from build123d import *

# Parameters (mm, degrees)
EXTRUDE_1_DEPTH     = 6
FILLET_1_R          = 0.5
SKETCH_2_W          = 0.4
SKETCH_2_H          = 0.4
EXTRUDE_2_DEPTH     = 2.5
SKETCH_3_W          = 0.8
SKETCH_3_H          = 5.4
CUT_EXTRUDE_1_DEPTH = 0.5
SKETCH_4_W          = 0.8
SKETCH_4_H          = 5.4
CUT_EXTRUDE_2_DEPTH = 0.5
SKETCH_5_W          = 0.5
SKETCH_5_H          = 4
CUT_EXTRUDE_3_DEPTH = 0.5
SKETCH_6_W          = 0.5
SKETCH_6_H          = 4
CUT_EXTRUDE_4_DEPTH = 0.5
SKETCH_7_R          = 0.35
EXTRUDE_3_DEPTH     = 0.7


with BuildPart() as part:
    # 草图1 → 凸台-拉伸1 (new body)
    with BuildSketch(Plane.XY):
        Polygon((-7, 5), (-2.5, 5), (-2.5, -2.5), (2.5, -2.5), (2.5, 5), (7, 5), (7, -5), (-7, -5), align=None)
    extrude(amount=EXTRUDE_1_DEPTH)

    # 圆角1
    fillet_1_edges = [part.edges().sort_by_distance(p)[0] for p in [
        (-2.5, 5, 3),
        (2.5, 5, 3),
    ]]
    fillet(fillet_1_edges, radius=FILLET_1_R)

    # 草图2 → 凸台-拉伸2 (add)
    with BuildSketch(Plane.XZ.offset(5)):
        with Locations((-5.15, 4.27)):
            Rectangle(SKETCH_2_W, SKETCH_2_H)
        with Locations((5.15, 4.27)):
            Rectangle(SKETCH_2_W, SKETCH_2_H)
        with Locations((-5.15, 1.73)):
            Rectangle(SKETCH_2_W, SKETCH_2_H)
        with Locations((5.15, 1.73)):
            Rectangle(SKETCH_2_W, SKETCH_2_H)
    extrude(amount=EXTRUDE_2_DEPTH)

    # 草图3 → 切除-拉伸1 (cut)
    with BuildSketch(Plane.ZY.offset(7)):
        with Locations((3.003385533, 2.3)):
            Rectangle(SKETCH_3_W, SKETCH_3_H)
    extrude(amount=-CUT_EXTRUDE_1_DEPTH, mode=Mode.SUBTRACT)

    # 草图4 → 切除-拉伸2 (cut)
    with BuildSketch(Plane(origin=(7, 0, 0), x_dir=(0, 0, -1), z_dir=(1, 0, 0))):
        with Locations((-3.003385533, 2.3)):
            Rectangle(SKETCH_4_W, SKETCH_4_H)
    extrude(amount=-CUT_EXTRUDE_2_DEPTH, mode=Mode.SUBTRACT)

    # 草图5 → 切除-拉伸3 (cut)
    with BuildSketch(Plane(origin=(-2.5, 0, 0), x_dir=(0, 0, -1), z_dir=(1, 0, 0))):
        with Locations((-3.003385533, 3)):
            Rectangle(SKETCH_5_W, SKETCH_5_H)
    extrude(amount=-CUT_EXTRUDE_3_DEPTH, mode=Mode.SUBTRACT)

    # 草图6 → 切除-拉伸4 (cut)
    with BuildSketch(Plane.ZY.offset(-2.5)):
        with Locations((3.003385533, 3)):
            Rectangle(SKETCH_6_W, SKETCH_6_H)
    extrude(amount=-CUT_EXTRUDE_4_DEPTH, mode=Mode.SUBTRACT)

    # 草图7 → 凸台-拉伸3 (add)
    with BuildSketch(Plane.XZ.offset(5)):
        with Locations(Location((-2.15, 5.65, 0), (0, 0, 90))):
            Circle(SKETCH_7_R)
        with Locations(Location((6.65, 0.35, 0), (0, 0, 270))):
            Circle(SKETCH_7_R)
    extrude(amount=EXTRUDE_3_DEPTH)


solid = part.part
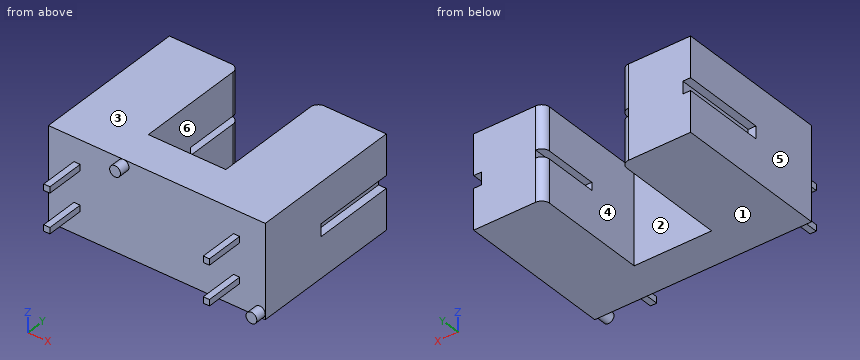
Design review of the part built by this model. Coordinates are the model's own, in mm. Face numbers are marked on the shaded views. A direction names the side the tool comes from. Round coordinates to 2 decimals unless told otherwise and drop trailing zeros. Order: outer loops, then holes, each group sorted by start corner. A loop starts at its lowest first (then second) coordinate and runs counter-clockwise, first axis right, second up.
1) Consider section D-D (x = 1). State the section outline as (y, z) points, plus the area to 3 significant figures.
The answers:
outline: (-5, 0) - (-2.5, 0) - (-2.5, 6) - (-5, 6) - close
area: 15.0 mm2
2) Draft analysis for pull direction X (two halves, no side actions). For the marked faces 3, 4, 5 and 6, state which applies: released by +X, released by -X, zero draft, split by the parting line, or undercut.
The answers:
face 3: zero draft
face 4: undercut
face 5: released by -X
face 6: undercut
3) For L1, parallel to X at y = -0.5, z = 5.1; L2, parallel to Y at x = -3, z = 0.95; L3, parallel to Y at x = -2, z = 1, list the stretches that pass through material, from the lowest coordinate up.
The answers:
L1: x = -7 to -2.5, 2.5 to 7
L2: y = -5 to 5
L3: y = -5 to -2.5
4) Machinability: for the marked faces 1 and 2, which of the approach directions +Z, -Z, +X, -X, +Y, -Y give a long, thin tool a straight path to every point of the face, cutting with its end or side? Answer none if there is none.
The answers:
face 1: -Z, +X, -X, +Y, -Y
face 2: +Z, -Z, +Y
5) Consider section C-C (y = 0.75). State the section outline as (x, z) points.
The answers:
outline: (-7, 0) - (-2.5, 0) - (-2.5, 6) - (-7, 6) - (-7, 3.4) - (-6.5, 3.4) - (-6.5, 2.6) - (-7, 2.6) - close; (2.5, 0) - (7, 0) - (7, 2.6) - (6.5, 2.6) - (6.5, 3.4) - (7, 3.4) - (7, 6) - (2.5, 6) - close
6) Clearance check with flat-ended pins moving along their axes: pin 1 Ø0.6 at (y, z) = (1.5, 3) entering from -X; pin 2 Ø2 at (x, z) = (-5.5, 5.5) entering from -Y; pin 3 Ø0.6 at (x, z) = (-7, 3) entering from +Y. State where each tip first meets the part, or that it passes through.
The answers:
pin 1: stops at x = -6.5
pin 2: stops at y = -5
pin 3: stops at y = -0.4
7) Consider section B-B (z = 2.1). State the section outline as (x, y) points, plus the area to 3 significant figures.
The answers:
outline: (-7, -5) - (7, -5) - (7, 5) - (3, 5) arc R0.5 ccw to (2.5, 4.5) - (2.5, -2.5) - (-2.5, -2.5) - (-2.5, 4.5) arc R0.5 ccw to (-3, 5) - (-7, 5) - close
area: 102 mm2
8) Consider section A-A (y = 3.25). State the section outline as (x, z) points.
The answers:
outline: (-7, 0) - (-2.5, 0) - (-2.5, 2.75) - (-3, 2.75) - (-3, 3.25) - (-2.5, 3.25) - (-2.5, 6) - (-7, 6) - (-7, 3.4) - (-6.5, 3.4) - (-6.5, 2.6) - (-7, 2.6) - close; (2.5, 0) - (7, 0) - (7, 2.6) - (6.5, 2.6) - (6.5, 3.4) - (7, 3.4) - (7, 6) - (2.5, 6) - (2.5, 3.25) - (3, 3.25) - (3, 2.75) - (2.5, 2.75) - close
